```python
from build123d import *

# Parameters (mm, degrees)
F2_R     = 5.025
F3_DEPTH = 25
F4_W     = 11
F4_H     = 20
F5_DEPTH = 20


with BuildPart() as f1:
    # F0 (on Front) → F1 (revolve)
    with BuildSketch(Plane.XZ):
        Polygon((15, 15), (0, 15), (0, -15), (15, -15), (15, 4.5), (13.5, 4.5), (13.5, 6), (15, 6), (15, 8), (13.5, 8), (13.5, 9.5), (15, 9.5), (15, 11.5), (13.5, 11.5), (13.5, 13), (15, 13), align=None)
    revolve(axis=Axis((0, 0, 0), (0, 0, -1)))

    # F2 (on Right) → F3 (cut, symmetric)
    with BuildSketch(Plane.YZ):
        with Locations((0, -5)):
            Circle(F2_R)
    extrude(amount=F3_DEPTH, both=True, mode=Mode.SUBTRACT)

    # F4 (on face) → F5 (cut)
    with BuildSketch(Plane(origin=(0, 0, -15), x_dir=(1, 0, 0), z_dir=(0, 0, -1))):
        Rectangle(F4_W, F4_H)
    extrude(amount=-F5_DEPTH, mode=Mode.SUBTRACT)


solid = f1.part
```
Check sheet for the modelled part. Datum: model origin and axes. Units: mm. A direction names the side the tool comes from. Coordinates: 2 decimals unless noted, no trailing zeros. Order: outer loops, then holes, each group sorted by start corner. A loop starts at its lowest first (then second) coordinate and runs counter-clockwise, first axis right, second up. Notation, with made-up numbers: M 17,11.25 L 34,11.25 A18 cw 34,26.25 Z; hole C 80,23 d11. An arc over 180 degrees is marked long. Write each question's results on one line, items separated by ' | '. Start each with the question number.
1. Material ranges on probe 1 along Z at (x, y) = (-12.25, 0) (3 decimals); probe 2 along Y at (x, z) = (0, 3.5); probe 3 along Z at (x, y) = (4.5, -7), recorded low to high.
2. Cross-section at A-A on z = 2. Record the cut outline in (x, y).
3. Go/stop test with flat-tipped pins: P1, Ø3.5, axis at x = 1.5, y = -4.5, coming from the -Z side; P2, Ø4, axis at y = 3, z = -7, coming from the -X side; P3, Ø1, axis at x = 12, z = 1, coming from the -Y side; P4, Ø9, axis at y = 0, z = -5, coming from the -X side. Record where each tip stops, or that it passes through.
4. Mould release check, pull along X, two halves, no side actions. Record for faces 4 (the face through (13.856, 5.745, -5.114)), 5 (the face through (-11.18, -7.85, 8)), 6 (the face through (0, -10, -5)): +X half, -X half, draft (parallel to the pull), parting line (faces both ways), or undercut.
5. Cross-section at C-C on z = -9. Record the cut outline in (x, y), and give its area (3 significant figures).
6. Access from +Z, -Z, +X, -X, +Y, -Y to the whole of each face (thin tool, end or side, straight path). Record for faces 1 (the face through (-5.5, 2, -10)), 2 (the face through (-2.93, 13.18, 8.76)), 3 (the face through (-14.985, -0.66, 7.014)).
Checks:
1) probe 1: z = -15 to -10.025, 0.025 to 15 | probe 2: y = -15 to -10, 10 to 15 | probe 3: z = 5 to 15
2) outline: C 0,0 d30; hole M -5.5,-10 L 5.5,-10 L 5.5,10 L -5.5,10 Z
3) P1: stops at z = 5 | P2: stops at x = -14.69 | P3: stops at y = -9.63 | P4: passes through
4) face 4: parting line | face 5: draft | face 6: undercut
5) outline: M -14.69,-3.04 A15 ccw 14.69,-3.04 L 5.5,-3.04 L 5.5,-10 L -5.5,-10 L -5.5,-3.04 Z; M -14.69,3.04 L -5.5,3.04 L -5.5,10 L 5.5,10 L 5.5,3.04 L 14.69,3.04 A15 ccw Z | area: 373 mm²
6) face 1: -Z | face 2: none | face 3: +Z, -Z
